Could you check a few things on this model? Use its own coordinates, in mm. A direction names the side the tool comes from. Round coordinates to 2 decimals unless told otherwise and drop trailing zeros. Order: outer loops, then holes, each group sorted by start corner. A loop starts at its lowest first (then second) coordinate and runs counter-clockwise, first axis right, second up. Notation, with made-up numbers: (-30.5, -4.5) - (28.5, -4.5) arc R23 cw to (28.5, 5.5) - close; hole circle Ø10 at (35.25, 17). An arc over 180 degrees is marked (long way). Return JSON: item names as keys, results as strings. Group by question number.
from build123d import *

# Parameters (mm, degrees)
SKETCH_1_W      = 60
SKETCH_1_H      = 40
EXTRUDE_1_DEPTH = 2
SKETCH_2_W      = 60
SKETCH_2_H      = 2
EXTRUDE_2_DEPTH = 30
SKETCH_3_W      = 60
SKETCH_3_H      = 2
EXTRUDE_3_DEPTH = 20


with BuildPart() as part:
    # 草图1 → 凸台-拉伸1 (new body)
    with BuildSketch(Plane.XY):
        with Locations((-1.578947368, -6.578947368)):
            Rectangle(SKETCH_1_W, SKETCH_1_H)
    extrude(amount=EXTRUDE_1_DEPTH)

    # 草图2 → 凸台-拉伸2 (add)
    with BuildSketch(Plane.XY.offset(2)):
        with Locations((-1.578947368, 12.421052632)):
            Rectangle(SKETCH_2_W, SKETCH_2_H)
        with Locations((-1.578947368, -25.578947368)):
            Rectangle(SKETCH_2_W, SKETCH_2_H)
    extrude(amount=EXTRUDE_2_DEPTH)

    # 草图3 → 凸台-拉伸3 (add)
    with BuildSketch(Plane(origin=(0, 0, 0), x_dir=(-1, 0, 0), z_dir=(0, 0, -1))):
        with Locations((1.578947368, 12.421052632)):
            Rectangle(SKETCH_3_W, SKETCH_3_H)
    extrude(amount=EXTRUDE_3_DEPTH)


solid = part.part
1) I want a section at B-B, the plane x = 10. List the corners of the cut face in (y, z) for me.
2) I want a section at D-D, the plane z = -16. List the corners of the cut face in (x, y) for me.
3) For faces 4 (the flat face through (-2, -26.579, 16)), 5 (the flat face through (-2, -7, 0)), 6 (the flat face through (-2, -6, 2)), which set-ups out of +Z, -Z, +X, -X, +Y, -Y let a thin tool reach every point of the face, with its end or its side?
4) If I drill on line 1 along Y through (x, z) = (9, 13.5); line 2 along Z through (x, y) = (15, 5.5); line 3 along Y through (x, z) = (9.5, -3), over which ranges is the centre line in solid material (lowest first)? Write a range as from..to.
5) Will these pins go through, and if not, where does the flat tip stop? pin 1 (11 mm diameter, centred on x = 8, y = -8.5, fed in from +Z); pin 2 (8 mm diameter, centred on y = -0.5, z = 9, fed in from -X); pin 3 (10 mm diameter, centred on x = 12, z = -8.5, fed in from -Y); pin 4 (10 mm diameter, centred on x = 9.5, y = -22, fed in from -Z).
6) We'd pull the mould along Y, two halves only. Please class faces 1 (the flat face through (-2, -26, 32)), 2 (the flat face through (-2, -24.579, 17)), 3 (the flat face through (-1, 11.421, -10)): +Y half, -Y half, draft (parallel to the pull), parting line (faces both ways), or undercut.
7) I want a section at C-C, the plane y = -3. List the corners of the cut face in (x, z) for me, plus the area to 3 significant figures.
8) I want a section at A-A, the plane z = 25.5. List the corners of the cut face in (x, y) for me.
Outcome:
{
 "1": {"outline": "(-26.58, 0) - (11.42, 0) - (11.42, -20) - (13.42, -20) - (13.42, 32) - (11.42, 32) - (11.42, 2) - (-24.58, 2) - (-24.58, 32) - (-26.58, 32) - close"},
 "2": {"outline": "(-31.58, 11.42) - (28.42, 11.42) - (28.42, 13.42) - (-31.58, 13.42) - close"},
 "3": {"face 4": "+Z, -Z, +X, -X, -Y", "face 5": "-Z, +X, -X, -Y", "face 6": "+Z, +X, -X"},
 "4": {"line 1": "-26.58..-24.58, 11.42..13.42", "line 2": "0..2", "line 3": "11.42..13.42"},
 "5": {"pin 1": "z = 2", "pin 2": "through", "pin 3": "y = 11.42", "pin 4": "z = 0"},
 "6": {"face 1": "draft", "face 2": "undercut", "face 3": "-Y half"},
 "7": {"outline": "(-31.58, 0) - (28.42, 0) - (28.42, 2) - (-31.58, 2) - close", "area": "120 mm^2"},
 "8": {"outline": "(-31.58, -26.58) - (28.42, -26.58) - (28.42, -24.58) - (-31.58, -24.58) - close; (-31.58, 11.42) - (28.42, 11.42) - (28.42, 13.42) - (-31.58, 13.42) - close"}
}
